Source: three-view drawing plus pictorial views. Frame: mm from the lowest corner of the part. A direction names the side the tool comes from. Round coordinates to 2 decimals unless told otherwise and drop trailing zeros. Loops run counter-clockwise (first coordinate to the right, second up) from the corner with the lowest first, then second, coordinate; pieces in that order, holes last. Notation, with made-up numbers: (8.5, 62) -> (58.5, 62) arc R23 cw to (58.5, 75) -> close; hole circle Ø4 at (78.25, -22.5). An arc over 180 degrees is marked (long way). Put each result on its own line as item: value. Start each with the question number.
1. Contact query for flat-ended pins moving along their axis: pin 1 (8 mm diameter, centred on x = 29.5, z = 1.5, fed in from +Y); pin 2 (1 mm diameter, centred on x = 22, z = 2, fed in from -Y); pin 3 (15 mm diameter, centred on x = 41.5, y = 18.5, fed in from +Z). Output: stop coordinate, or through.
2. Cut plane B-B (y = 19). Return the cut outline in (x, z), then the cut area to 3 significant figures.
3. Cut plane D-D (x = 19). Return the cut outline in (y, z).
4. Draft query along Y for the marked faces 3, 4 and 5. Return one class per face: pulls with the +Y half, pulls with the -Y half, needs draft (parallel to the pull), parting line crosses it, or undercut.
5. Material intervals for L1, parallel to Y at x = 43.5, z = 12.75; L2, parallel to X at y = 13.5, z = 10; L3, parallel to Z at x = 9, y = 11, sorted ascending.
6. Cut plane C-C (z = 2). Return the cut outline in (x, y).
7. Set-up query: the marked faces 1 and 2. Return all of +Z, -Z, +X, -X, +Y, -Y with unobstructed straight access to the full face (end or side cutting, diameter ignored); none if empty.
8. Cut plane A-A (z = 12.5). Return the cut outline in (x, y).
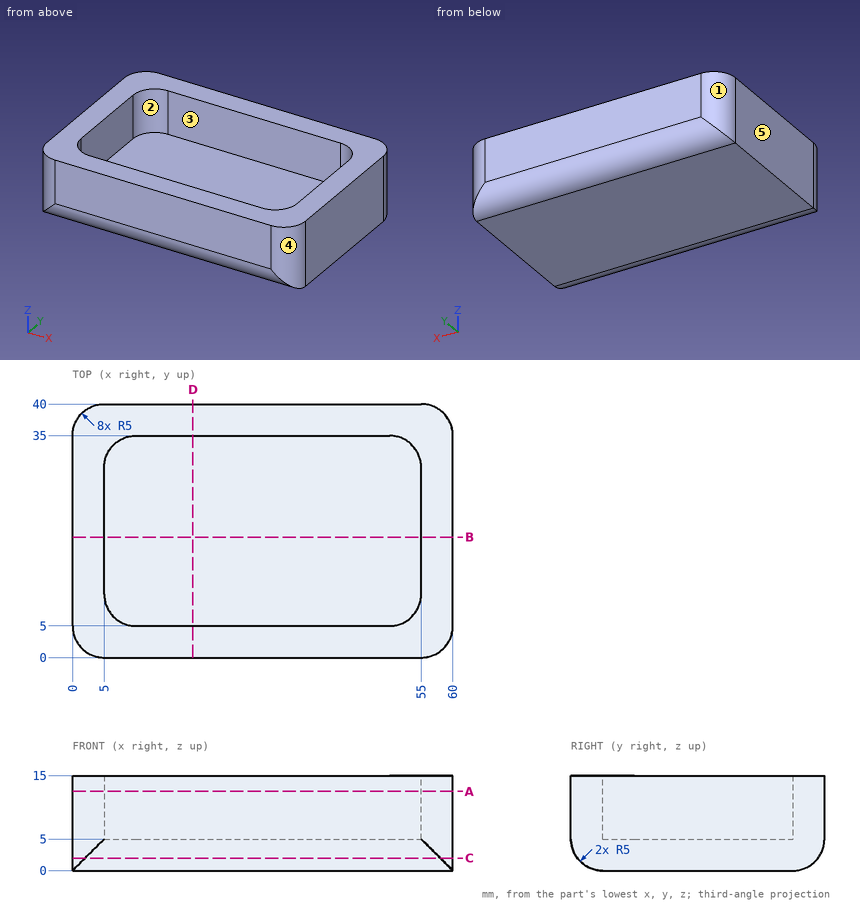
Solution:
1. pin 1: stops at y = 40
1. pin 2: stops at y = 0.67
1. pin 3: stops at z = 5
2. outline: (0, 0) -> (60, 0) -> (60, 15) -> (55, 15) -> (55, 5) -> (5, 5) -> (5, 15) -> (0, 15) -> close
2. area: 400 mm^2
3. outline: (0, 5) arc R5 ccw to (5, 0) -> (35, 0) arc R5 ccw to (40, 5) -> (40, 15) -> (35, 15) -> (35, 5) -> (5, 5) -> (5, 15) -> (0, 15) -> close
4. face 3: undercut
4. face 4: pulls with the -Y half
4. face 5: needs draft
5. L1: y = 0 to 5, 35 to 40
5. L2: x = 0 to 5, 55 to 60
5. L3: z = 0 to 5
6. outline: (0, 5) arc R5 ccw to (2, 1) -> (58, 1) arc R5 ccw to (60, 5) -> (60, 35) arc R5 ccw to (58, 39) -> (2, 39) arc R5 ccw to (0, 35) -> close
7. face 1: +Z, -Z, -X, +Y
7. face 2: +Z
8. outline: (0, 5) arc R5 ccw to (5, 0) -> (55, 0) arc R5 ccw to (60, 5) -> (60, 35) arc R5 ccw to (55, 40) -> (5, 40) arc R5 ccw to (0, 35) -> close; hole (5, 10) arc R5 ccw to (10, 5) -> (50, 5) arc R5 ccw to (55, 10) -> (55, 30) arc R5 ccw to (50, 35) -> (10, 35) arc R5 ccw to (5, 30) -> close
